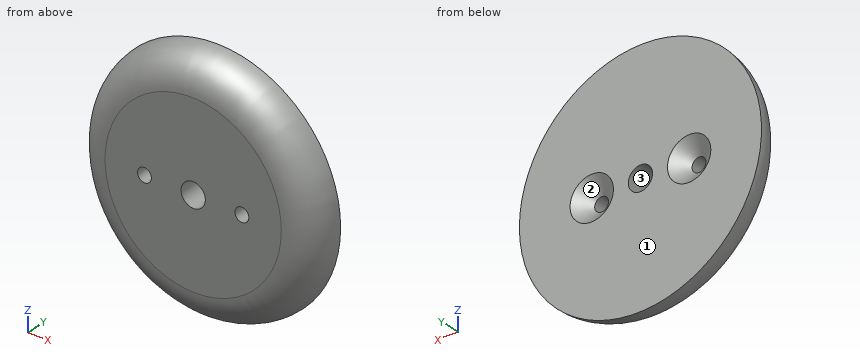
```python
from build123d import *

# Parameters (mm, degrees)
F0_R           = 69.8
F0_R_2         = 5
F1_DEPTH       = 19
F2_R           = 18.99999
F3_D           = 14
F3_DEPTH       = 20
F3_TIP         = 4.2060243332
F4_D           = 8
F4_DEPTH       = 20
F4_CSINK_D     = 25
F4_CSINK_ANGLE = 100
F4_TIP         = 2.4034424761


# Not quite as in the source:
# - a fillet or chamfer is up to 0.001 mm smaller than in the source, because OpenCascade refuses the exact size


with BuildPart() as f1:
    # F0 (on Front) → F1 (new body)
    with BuildSketch(Plane.XZ):
        Circle(F0_R)
        with Locations((-28.077211231, 0)):
            Circle(F0_R_2, mode=Mode.SUBTRACT)
        with Locations((28.077211231, 0)):
            Circle(F0_R_2, mode=Mode.SUBTRACT)
        with Locations((-28.077211231, 0)):
            Circle(F0_R_2)
        with Locations((28.077211231, 0)):
            Circle(F0_R_2)
    extrude(amount=F1_DEPTH)

    # F2 (radius 19 in the source; OpenCascade refuses exactly that, so slightly less here)
    f2_edges = [f1.edges().sort_by_distance(p)[0] for p in [
        (-69.8, -19, 0),
    ]]
    fillet(f2_edges, radius=F2_R)

    # F3
    with Locations(Plane(origin=(0, 0, 0), x_dir=(1, 0, 0), z_dir=(0, 1, 0))):
        with Locations((0, 0)):
            Hole(F3_D / 2, depth=F3_DEPTH)
            with Locations((0, 0, -(F3_DEPTH + F3_TIP / 2))):  # 118° drill point
                Cone(0, F3_D / 2, F3_TIP, mode=Mode.SUBTRACT)

    # F4
    with Locations(Plane(origin=(0, 0, 0), x_dir=(1, 0, 0), z_dir=(0, 1, 0))):
        with Locations((28.077211231, 0), (-28.077211231, 0)):
            CounterSinkHole(F4_D / 2, F4_CSINK_D / 2, depth=F4_DEPTH, counter_sink_angle=F4_CSINK_ANGLE)
            with Locations((0, 0, -(F4_DEPTH + F4_TIP / 2))):  # 118° drill point
                Cone(0, F4_D / 2, F4_TIP, mode=Mode.SUBTRACT)


solid = f1.part
```
Source: CAD feature listing. Evaluate the final solid. Frame: model axes, mm. Face numbers are marked on the shaded views. Coordinates: 2 decimals unless noted, no trailing zeros. Write each loop counter-clockwise with the first axis right and the second up, starting at its lowest first coordinate (ties: lowest second). Pieces come first, ordered by that corner, then holes. Notation, with made-up numbers: M -22,42.5 L -11,42.5 A21 cw -11,74.5 Z; hole C 1.25,1 d2. An arc over 180 degrees is marked long. Answer as a JSON object with one key per item and string values.
1. Cut plane C-C on y = -9.25. Output: boundary loops of the cut face in (x, z), plus the area to 3 significant figures.
Evaluation:
{"outline": "C 0,0 d134.79; hole C -28.08,0 d8; hole C 0,0 d14; hole C 28.08,0 d8", "area": "14,000 mm^2"}
2. Cut plane A-A on z = 0. State how many separate pieces and enclosed holes the cut face has, plus the area to 3 significant figures.
Evaluation:
{"separate pieces": "4", "enclosed holes": "0", "area": "1,810 mm^2"}
3. Draft query along X for the marked faces 1, 2 and 3. Return one class per face: released by +X, released by -X, zero draft, split by the parting line, or undercut.
Evaluation:
{"face 1": "zero draft", "face 2": "undercut", "face 3": "undercut"}
4. Ray query, L1, parallel to X at y = -10, z = 5; L2, parallel to Z at x = -31, y = -11; L3, parallel to Z at x = -29, y = -8.75. Return the intervals inside material, ascending.
Evaluation:
{"L1": "-66.77 to -4.9, 4.9 to 66.77", "L2": "-58.6 to -2.73, 2.73 to 58.6", "L3": "-61.14 to -3.89, 3.89 to 61.14"}
5. Contact query for flat-ended pins moving along their axis: P1, Ø2, axis at x = 49.5, y = -3.5, coming from the -Z side; P2, Ø4, axis at y = -12, z = 25.5, coming from the +X side; P3, Ø6, axis at x = -33, y = -13.5, coming from the +Z side; P4, Ø6.5, axis at x = 28.08, z = 0, coming from the -Y side. Output: stop coordinate, or through.
Evaluation:
{"P1": "z = -49.78", "P2": "x = 62.13", "P3": "z = 58.42", "P4": "through"}
6. Cut plane D-D on y = -1.75. Output: boundary loops of the cut face in (x, z).
Evaluation:
{"outline": "C 0,0 d139.44; hole C -28.08,0 d20.83; hole C 0,0 d14; hole C 28.08,0 d20.83"}
